```python
from build123d import *

# Parameters (mm, degrees)
SKETCH1_W           = 101.6
SKETCH1_H           = 19.05
BOSS_EXTRUDE1_DEPTH = 3.175
SKETCH2_W           = 3.048
SKETCH2_H           = 7.62
CUT_EXTRUDE1_DEPTH  = 4.175
SKETCH3_W           = 5.7
SKETCH3_H           = 10
CUT_EXTRUDE2_DEPTH  = 4.175
CHAMFER1_SIZE       = 1


with BuildPart() as part:
    # Sketch1 → Boss-Extrude1 (new body)
    with BuildSketch(Plane.XY):
        with Locations((50.8, 9.525)):
            Rectangle(SKETCH1_W, SKETCH1_H)
    extrude(amount=BOSS_EXTRUDE1_DEPTH)

    # Sketch2 → Cut-Extrude1 (cut, through all)
    with BuildSketch(Plane.XY.offset(3.175)):
        with Locations((9.892117884, 9.525)):
            Rectangle(SKETCH2_W, SKETCH2_H)
        with Locations((91.707882116, 9.525)):
            Rectangle(SKETCH2_W, SKETCH2_H)
    extrude(amount=-CUT_EXTRUDE1_DEPTH, mode=Mode.SUBTRACT)

    # Sketch3 → Cut-Extrude2 (cut, through all)
    with BuildSketch(Plane.XY.offset(3.175)):
        with Locations((37.95, 9.525)):
            Rectangle(SKETCH3_W, SKETCH3_H)
        with Locations((63.65, 9.525)):
            Rectangle(SKETCH3_W, SKETCH3_H)
        with Locations((79.35, 9.525)):
            Rectangle(SKETCH3_W, SKETCH3_H)
        with Locations((22.25, 9.525)):
            Rectangle(SKETCH3_W, SKETCH3_H)
    extrude(amount=-CUT_EXTRUDE2_DEPTH, mode=Mode.SUBTRACT)

    # Chamfer1
    chamfer1_edges = [part.edges().sort_by_distance(p)[0] for p in [
        (76.5, 14.525, 1.5875),
        (82.2, 14.525, 1.5875),
        (19.4, 14.525, 1.5875),
        (25.1, 14.525, 1.5875),
        (60.8, 14.525, 1.5875),
        (66.5, 14.525, 1.5875),
        (35.1, 14.525, 1.5875),
        (40.8, 14.525, 1.5875),
    ]]
    chamfer(chamfer1_edges, length=CHAMFER1_SIZE)


solid = part.part
```
The listing builds one solid part. Answer for the finished solid, in the listing's coordinates (mm). A direction names the side the tool comes from. Give positions to 0.01 mm unless a question says otherwise; leave off trailing zeros. Order: outer loops, then holes, each group sorted by start corner. A loop starts at its lowest first (then second) coordinate and runs counter-clockwise, first axis right, second up. Notation, with made-up numbers: (35, -2) -> (55, -2) arc R15 cw to (55, 11) -> close; hole circle Ø9 at (-16, -25). An arc over 180 degrees is marked (long way). Answer as a JSON object with one key per item and string values. Group by question number.
Item 1: The part is cut by section B-B on y = 6.75. Write down the section's boundary in (x, z) (3 decimals).
Item 2: Consider L1, parallel to X at y = 5.25, z = 2.35; L2, parallel to Y at x = 65, z = 0.8 (3 decimals); L3, parallel to X at y = 14.25, z = 0.5 (3 decimals). Determine where each line is inside the solid, lowest interval first. Write a range as from..to.
Item 3: A tool of negligible diameter and unlimited length cuts with its end or side. For faces 4 (the flat face through (35.1, 9, 2)), 5 (the flat face through (50, 19.05, 2)), from which of +Z, -Z, +X, -X, +Y, -Y can it reach the whole face along a straight path? Write none if from no direction.
Item 4: Determine the mould class of faces 1 (the flat face through (79, 14.525, 2)), 2 (the flat face through (0, 9, 2)), 3 (the flat face through (50, 0, 2)) for opening direction Y: pulls with the +Y half, pulls with the -Y half, needs draft (parallel to the pull), parting line crosses it, or undercut.
Item 5: The part is cut by section C-C on z = 1.4. Give the number of separate pieces and of enclosed holes in the cut face, and give its area (3 significant figures).
Item 6: The part is cut by section A-A on x = 37. Write down the section's boundary in (y, z) (3 decimals).
Result set:
{
 "1": {"outline": "(0, 0) -> (8.368, 0) -> (8.368, 3.175) -> (0, 3.175) -> close; (11.416, 0) -> (19.4, 0) -> (19.4, 3.175) -> (11.416, 3.175) -> close; (25.1, 0) -> (35.1, 0) -> (35.1, 3.175) -> (25.1, 3.175) -> close; (40.8, 0) -> (60.8, 0) -> (60.8, 3.175) -> (40.8, 3.175) -> close; (66.5, 0) -> (76.5, 0) -> (76.5, 3.175) -> (66.5, 3.175) -> close; (82.2, 0) -> (90.184, 0) -> (90.184, 3.175) -> (82.2, 3.175) -> close; (93.232, 0) -> (101.6, 0) -> (101.6, 3.175) -> (93.232, 3.175) -> close"},
 "2": {"L1": "0..19.4, 25.1..35.1, 40.8..60.8, 66.5..76.5, 82.2..101.6", "L2": "0..4.525, 14.525..19.05", "L3": "0..20.125, 24.375..35.825, 40.075..61.525, 65.775..77.225, 81.475..101.6"},
 "3": {"face 4": "+Z, -Z", "face 5": "+Z, -Z, +X, -X, +Y"},
 "4": {"face 1": "undercut", "face 2": "needs draft", "face 3": "pulls with the -Y half"},
 "5": {"separate pieces": "1", "enclosed holes": "6", "area": "1,670 mm²"},
 "6": {"outline": "(0, 0) -> (4.525, 0) -> (4.525, 3.175) -> (0, 3.175) -> close; (14.525, 0) -> (19.05, 0) -> (19.05, 3.175) -> (14.525, 3.175) -> close"}
}
